from build123d import *

# Parameters (mm, degrees)
MOTOR_RING_DEPTH      = 12.5
MOTOR_RING_DEPTH_BACK = 6
SKETCH1_R             = 35
SKETCH1_R_2           = 32
SKETCH3_R             = 35
SKETCH3_R_2           = 6
MOTOR_CAP_DEPTH       = 3
BULK_START            = 3
SKETCH2_R             = 32
BULK_EXTRUDE_DEPTH    = 3
FILLET2_R             = 10
FILLET3_R             = 10
FILLET4_R             = 3
FILLET5_R             = 1


with BuildPart() as part:
    # Sketch1 → MOTOR RING (new, two sides: drawn at the far end of the back side and taken through both)
    with BuildSketch(Plane(origin=(-42.5, 0, 0), x_dir=(0, 0, -1), z_dir=(1, 0, 0)).offset(-MOTOR_RING_DEPTH_BACK)):
        with Locations(Location((50, -18.372727273, 0), (0, 0, 270))):
            Circle(SKETCH1_R)
        with Locations(Location((50, -18.372727273, 0), (0, 0, 270))):
            Circle(SKETCH1_R_2, mode=Mode.SUBTRACT)
    extrude(amount=MOTOR_RING_DEPTH + MOTOR_RING_DEPTH_BACK)

    # Sketch3 → MOTOR CAP (add)
    with BuildSketch(Plane(origin=(-48.5, 0, 0), x_dir=(0, 0, -1), z_dir=(1, 0, 0))):
        with Locations(Location((50, -18.372727273, 0), (0, 0, 270))):
            Circle(SKETCH3_R)
        with Locations(Location((50, -18.372727273, 0), (0, 0, 90))):
            Circle(SKETCH3_R_2, mode=Mode.SUBTRACT)
    extrude(amount=-MOTOR_CAP_DEPTH)

    # Sketch2 → BULK EXTRUDE (add)
    with BuildSketch(Plane.ZY.offset(27).offset(BULK_START)):
        with BuildLine():
            Line((-105, -18.372727273), (-105, 69.627272727))
            Line((-105, 69.627272727), (5, 69.627272727))
            Line((5, 69.627272727), (5, -18.372727273))
            ThreePointArc((5, -18.372727273), (-50, -73.372727273), (-105, -18.372727273))
        make_face()
        with Locations(Location((-50, -18.372727273, 0), (0, 0, 270))):
            Circle(SKETCH2_R, mode=Mode.SUBTRACT)
    extrude(amount=BULK_EXTRUDE_DEPTH)

    # Fillet2
    # the kernel refuses this fillet: 10 mm, written as the material it adds along each edge
    with BuildSketch(Plane(origin=(-33, -18.372727273, -50), x_dir=(0, -1, 0), z_dir=(0, 0, -1))) as fillet2_piece_1:
        with BuildLine():
            CenterArc((35 + FILLET2_R, FILLET2_R), FILLET2_R, 180, 90)
            Line((35 + FILLET2_R, 0), (35, 0))
            Line((35, 0), (35, FILLET2_R))
        make_face()
    revolve(axis=Axis((-33, -18.372727273, -50), (-1, 0, 0)))

    # Fillet3
    fillet3_edges = [part.edges().sort_by_distance(p)[0] for p in [
        (-30, 13.627272727, -50),
    ]]
    fillet(fillet3_edges, radius=FILLET3_R)

    # Fillet4
    fillet4_edges = [part.edges().sort_by_distance(p)[0] for p in [
        (-51.5, 16.627272727, -50),
    ]]
    fillet(fillet4_edges, radius=FILLET4_R)

    # Fillet5
    fillet5_edges = [part.edges().sort_by_distance(p)[0] for p in [
        (-48.5, 13.627272727, -50),
    ]]
    fillet(fillet5_edges, radius=FILLET5_R)


solid = part.part
Geometry check sheet. Reference: the model listing, model coordinates, mm. A direction names the side the tool comes from. Round coordinates to 2 decimals unless told otherwise and drop trailing zeros. Order: outer loops, then holes, each group sorted by start corner. A loop starts at its lowest first (then second) coordinate and runs counter-clockwise, first axis right, second up. Notation, with made-up numbers: M 43,-18 L 93,-18 A22 ccw 93,9 Z; hole C -29,60.25 d11. An arc over 180 degrees is marked long. Answer in a Markdown table with one row per item.
(1) Draft check along Z on faces 4 (the face through (-49.979, -24.367, -49.736)), 5 (the face through (-31, 26, 5)), 6 (the face through (-33, 31, -49)). Enter one of: released by +Z, released by -Z, zero draft, split by the parting line, or undercut.
Responses:
| item | result |
|---|---|
| face 4 | undercut |
| face 5 | released by +Z |
| face 6 | zero draft |
(2) Sectioned sample at A-A, the plane z = -50. Record the cut outline in (x, y).
Responses:
| item | result |
|---|---|
| outline | M -51.5,-50.37 A3 ccw -48.5,-53.37 L -43,-53.37 A10 cw -33,-63.37 L -33,-73.37 L -30,-73.37 L -30,-60.37 A10 ccw -40,-50.37 L -47.5,-50.37 A1 cw -48.5,-49.37 L -48.5,-24.37 L -51.5,-24.37 Z; M -51.5,-12.37 L -48.5,-12.37 L -48.5,12.63 A1 cw -47.5,13.63 L -40,13.63 A10 ccw -30,23.63 L -30,69.63 L -33,69.63 L -33,26.63 A10 cw -43,16.63 L -48.5,16.63 A3 ccw -51.5,13.63 Z |
(3) Scan lines: probe 1 along X at (y, z) = (-27, -28); probe 2 along X at (y, z) = (25, -11); probe 3 along Z at (x, y) = (-37.5, -22.5). Record each from-to range of solid material in increasing order. Write a range as from..to.
Responses:
| item | result |
|---|---|
| probe 1 | x = -51.5..-48.5 |
| probe 2 | x = -33..-30 |
| probe 3 | z = -86.42..-82.05, -17.95..-13.58 |
(4) Sectioned sample at B-B, the plane x = -46. Record the cut outline in (y, z).
Responses:
| item | result |
|---|---|
| outline | C -18.37,-50 d70; hole C -18.37,-50 d64 |
(5) Tool access check on faces 1 (the face through (-48.5, -17.9, -43.5)), 2 (the face through (-31, 25, -105)), 3 (the face through (-45.7, -13.8, -84.7)). Record the directions out of +Z, -Z, +X, -X, +Y, -Y that give a thin tool (end or side, any length) a straight path to the whole face; none if there is none.
Responses:
| item | result |
|---|---|
| face 1 | +X |
| face 2 | -Z, +X, -X, +Y, -Y |
| face 3 | -X |
(6) Sectioned sample at D-D, the plane x = -36.5. Record the cut outline in (y, z) (1 decimal).
Responses:
| item | result |
|---|---|
| outline | C -18.4,-50 d74.8; hole C -18.4,-50 d65.3 |
(7) Go/stop test with flat-tipped pins: P1, Ø2, axis at x = -39.5, z = -20, coming from the +Y side; P2, Ø12, axis at x = -40.5, y = -21, coming from the -Z side; P3, Ø10, axis at x = -33, z = -89, coming from the -Y side. Record where each tip stops, or that it passes through.
Responses:
| item | result |
|---|---|
| P1 | stops at y = 2.49 |
| P2 | stops at z = -89.65 |
| P3 | stops at y = -61.6 |
(8) Sectioned sample at C-C, the plane y = 46.5. Record the cut outline in (x, z).
Responses:
| item | result |
|---|---|
| outline | M -33,-105 L -30,-105 L -30,5 L -33,5 Z |
